Answer from the drawing. Dimensions are ordinates in mm from the lowest x, y and z of the part. A direction names the side the tool comes from. Coordinates: 2 decimals unless noted, no trailing zeros. Loops run counter-clockwise (first coordinate to the right, second up) from the corner with the lowest first, then second, coordinate; pieces in that order, holes last. Notation, with made-up numbers: (-37, -37.75) - (-14, -37.75) arc R28 ccw to (-14, -13.75) - close; hole circle Ø10 at (-15, 32.5). An arc over 180 degrees is marked (long way). One line per question, with ' | ' between items. Start each with the question number.
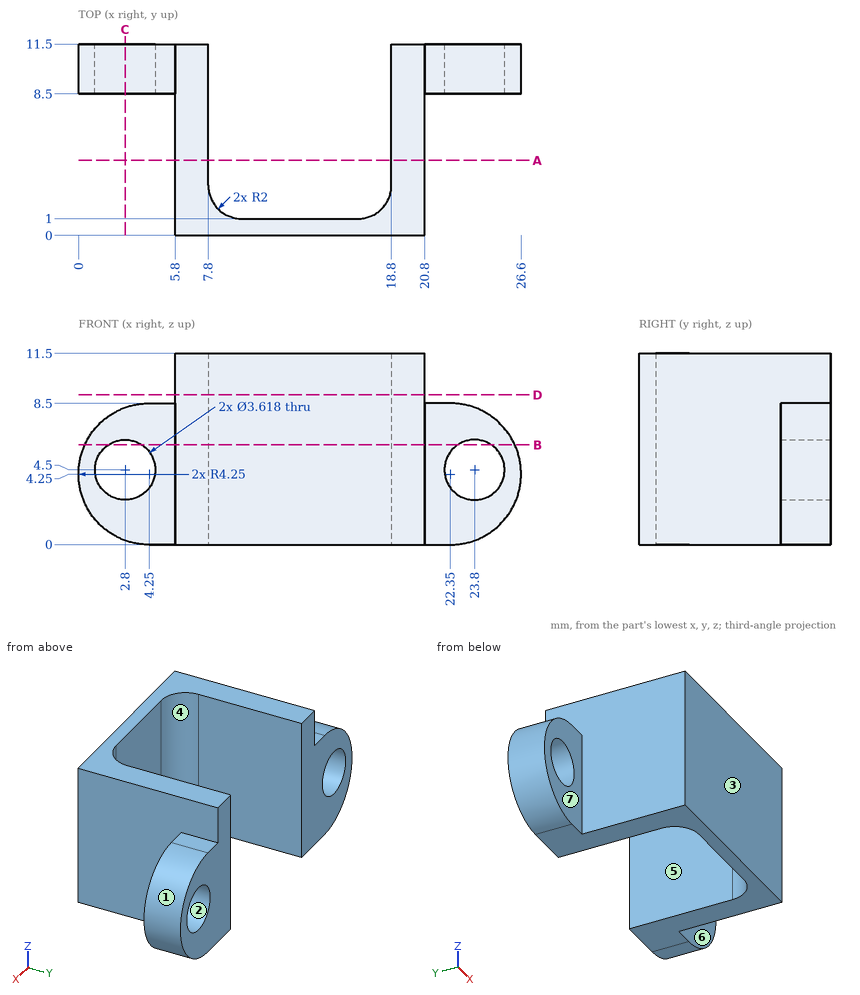
1) The part is cut by section C-C on x = 2.8. Write down the section's boundary in (y, z) (1 decimal).
2) Find the intervals of material crossed by line 1 along X through (y, z) = (3.5, 1.25); line 2 along X through (y, z) = (10.5, 3.5) (1 decimal); line 3 along X through (y, z) = (9.8, 4.5), in increasing order. Write a range as from..to.
3) Which of the six approach directions +Z, -Z, +X, -X, +Y, -Y give full straight-line access (tool end or side, diameter ignored) to the marked faces 5, 6 and 7?
4) The part is cut by section D-D on z = 9. Write down the section's boundary in (x, y).
5) The part is cut by section B-B on z = 6. Write down the section's boundary in (x, y).
6) The mould has two halves that part along X. Classify the marked faces 1, 2, 3 and 4: released by +X, released by -X, zero draft, split by the parting line, or undercut.
7) The part is cut by section A-A on y = 4.5. Write down the section's boundary in (x, z), and give its area (3 significant figures).
8) Given pin 1 Ø0.8 at (x, y) = (5, 10) entering from +Z; pin 2 Ø4 at (y, z) = (1.5, 9) entering from -X; pin 3 Ø3.5 at (x, z) = (2.8, 4.5) entering from -Y; pin 4 Ø6 at (y, z) = (2, 8.5) entering from +X, each flat-ended and moving along its own axis, determine where each tip first touches the part or whether it passes through.
Answer below:
1) outline: (8.5, 0.3) - (11.5, 0.3) - (11.5, 2.7) - (8.5, 2.7) - close; (8.5, 6.3) - (11.5, 6.3) - (11.5, 8.2) - (8.5, 8.2) - close
2) line 1: 5.8..7.8, 18.8..20.8 | line 2: 0.1..1.3, 4.3..7.8, 18.8..22.3, 25.3..26.5 | line 3: 0.01..0.99, 4.61..7.8, 18.8..21.99, 25.61..26.59
3) face 5: +Z, -Z, +Y | face 6: +Z, -Z, +X, -Y | face 7: +Z, -Z, -X, -Y
4) outline: (5.8, 0) - (20.8, 0) - (20.8, 11.5) - (18.8, 11.5) - (18.8, 3) arc R2 cw to (16.8, 1) - (9.8, 1) arc R2 cw to (7.8, 3) - (7.8, 11.5) - (5.8, 11.5) - close
5) outline: (0.38, 8.5) - (1.79, 8.5) - (1.79, 11.5) - (0.38, 11.5) - close; (3.81, 8.5) - (5.8, 8.5) - (5.8, 0) - (20.8, 0) - (20.8, 8.5) - (22.79, 8.5) - (22.79, 11.5) - (18.8, 11.5) - (18.8, 3) arc R2 cw to (16.8, 1) - (9.8, 1) arc R2 cw to (7.8, 3) - (7.8, 11.5) - (3.81, 11.5) - close; (24.81, 8.5) - (26.22, 8.5) - (26.22, 11.5) - (24.81, 11.5) - close
6) face 1: released by +X | face 2: undercut | face 3: zero draft | face 4: undercut
7) outline: (5.8, 0) - (7.8, 0) - (7.8, 11.5) - (5.8, 11.5) - close; (18.8, 0) - (20.8, 0) - (20.8, 11.5) - (18.8, 11.5) - close | area: 46.0 mm2
8) pin 1: z = 8.5 | pin 2: x = 5.8 | pin 3: through | pin 4: x = 20.8
